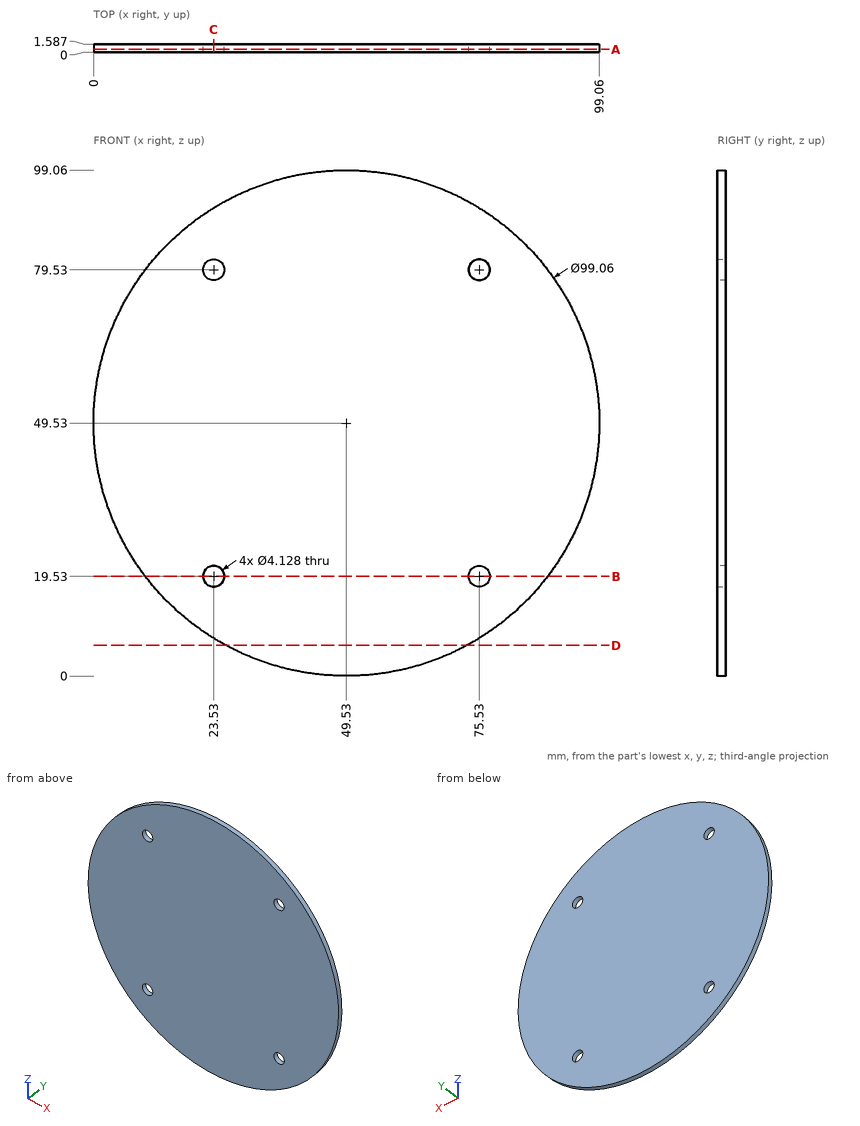
Print and shaded views of the part. All mm, measured from the part's lowest x, y and z. Give positions to 0.01 mm unless a question says otherwise; leave off trailing zeros. Loops run counter-clockwise (first coordinate to the right, second up) from the corner with the lowest first, then second, coordinate; pieces in that order, holes last.
1) Saw through at B-B (z = 19.53). Write the cut outline in (x, y), plus the area to 3 significant figures.
2) Wall check: line 1 (X direction, y = 1, z = 19.53) (1 decimal); line 2 (Z direction, x = 23.53, y = 0.45) (1 decimal); line 3 (X direction, y = 1.1, z = 20.5). Give the ranges that are in metal, low to high.
3) Saw through at A-A (y = 0.55). Write the cut outline in (x, z), plus the area to 3 significant figures.
4) Saw through at C-C (x = 23.53). Write the cut outline in (y, z).
5) Saw through at D-D (z = 6). Write the cut outline in (x, y).
Answer block:
1. outline: (10.12, 0) - (21.47, 0) - (21.47, 1.59) - (10.12, 1.59) - close; (25.59, 0) - (73.47, 0) - (73.47, 1.59) - (25.59, 1.59) - close; (77.59, 0) - (88.94, 0) - (88.94, 1.59) - (77.59, 1.59) - close
1. area: 112 mm2
2. line 1: x = 10.1 to 21.5, 25.6 to 73.5, 77.6 to 88.9
2. line 2: z = 7.4 to 17.5, 21.6 to 77.5, 81.6 to 91.7
2. line 3: x = 9.4 to 21.71, 25.35 to 73.71, 77.35 to 89.66
3. outline: circle Ø99.06 at (49.53, 49.53); hole circle Ø4.13 at (23.53, 19.53); hole circle Ø4.13 at (23.53, 79.53); hole circle Ø4.13 at (75.53, 19.53); hole circle Ø4.13 at (75.53, 79.53)
3. area: 7,650 mm2
4. outline: (0, 7.37) - (1.59, 7.37) - (1.59, 17.47) - (0, 17.47) - close; (0, 21.59) - (1.59, 21.59) - (1.59, 77.47) - (0, 77.47) - close; (0, 81.59) - (1.59, 81.59) - (1.59, 91.69) - (0, 91.69) - close
5. outline: (25.9, 0) - (73.16, 0) - (73.16, 1.59) - (25.9, 1.59) - close
